The listing builds one solid part. Answer for the finished solid, in the listing's coordinates (mm). A direction names the side the tool comes from. Give positions to 0.01 mm unless a question says otherwise; leave off trailing zeros. Loops run counter-clockwise (first coordinate to the right, second up) from the corner with the lowest first, then second, coordinate; pieces in that order, holes last. Notation, with made-up numbers: M -9.75,84 L 22.25,84 A13 ccw 22.25,94 Z; hole C 43.25,-14 d10. An arc over 180 degrees is marked long. Return JSON: item names as keys, results as strings.
Autodesk Inventor part; units mm, degrees
ref_plane "YZ Plane" through (0, 0, 0) normal (1, 0, 0) x (0, 1, 0)
ref_plane "XZ Plane" through (0, 0, 0) normal (0, 1, 0) x (-1, 0, 0)
ref_plane "XY Plane" through (0, 0, 0) normal (0, 0, 1) x (1, 0, 0)
sketch "Sketch4" plane through (0, 0, 0) normal (0, 1, 0) x (-1, 0, 0)
  line L0 (0, 0) -> (13, 0)
  line L1 (13, 0) -> (13, -13)
  line L2 (13, -13) -> (8.925, -13)
  line L3 (8.925, -13) -> (8.925, -22.5)
  line L4 (8.925, -22.5) -> (1.425, -22.5)
  line L5 (1.425, -22.5) -> (1.425, -13)
  line L6 (1.425, -13) -> (0, -13)
  line L7 (0, -13) -> (0, 0)
  dimension "d17" = 13
  dimension "d18" = 13
  dimension "d19" = 7.5
  dimension "d20" = 1.425
  dimension "d21" = 9.5
extrude "Extrusion2" add sketch "Sketch4" along normal blind 8
sketch "Sketch5" plane through (0, 8, 0) normal (0, 1, 0) x (1, 0, 0)
  line L0 (-8.925, 15) -> (-6.425, 15)
  line L1 (-6.425, 15) -> (-6.425, 20.5)
  line L2 (-6.425, 20.5) -> (-8.925, 20.5)
  line L3 (-8.925, 20.5) -> (-8.925, 15)
  line L4 (-1.425, 22.5) -> (-8.925, 22.5)
  line L5 (-8.925, 22.5) -> (-8.925, 13)
  point P0 (0, 0)
  dimension "d24" = 5.5
  dimension "d25" = 2.5
  dimension "d26" = 2
extrude "Extrusion3" cut sketch "Sketch5" against normal through all
sketch "Sketch6" plane through (0, 8, 0) normal (0, 1, 0) x (1, 0, 0)
  circle A0 centre (-6.5, 6.5) radius 4
  line L0 (-13, 0) -> (0, 0)
  line L1 (0, 0) -> (0, 13)
  dimension "d29" = 8
  dimension "d30" = 6.5
  dimension "d31" = 6.5
extrude "Extrusion4" cut sketch "Sketch6" against normal through all
sketch "Sketch7" plane through (0, 8, 0) normal (0, 1, 0) x (1, 0, 0)
  line L0 (-4.425, 8.5) -> (-3.425, 8.5)
  line L1 (-3.425, 8.5) -> (-3.425, 22.5)
  line L2 (-3.425, 22.5) -> (-4.425, 22.5)
  line L3 (-4.425, 22.5) -> (-4.425, 8.5)
  line L4 (-1.425, 22.5) -> (-8.925, 22.5)
  line L5 (-1.425, 13) -> (-1.425, 22.5)
  point P0 (0, 0)
  dimension "d34" = 1
  dimension "d35" = 14
  dimension "d36" = 2
extrude "Extrusion5" cut sketch "Sketch7" against normal through all
sketch "Sketch8" plane through (-1.425, 0, -13) normal (1, 0, 0) x (0, 0, -1)
  circle A0 centre (4.75, 4) radius 1.65
  line L0 (0, 0) -> (9.5, 0)
  line L1 (9.5, 0) -> (9.5, 8)
  point P0 (-13, 0)
  dimension "d39" = 3.3
  dimension "d40" = 4
  dimension "d41" = 4.75
extrude "Extrusion6" cut sketch "Sketch8" against normal through all
fillet "Fillet1" radius 2 4 edges at (-13, 4, -13) (-13, 4, 0) (0, 4, 0) (0, 4, -13)
properties part number "COLLIER"
(1) Straight lines are drawn through the part: line 1 along Z through (x, y) = (-6.5, 1); line 2 along Y through (x, z) = (-5.1, -17.75); line 3 along X through (y, z) = (3.5, -10.75) (3 decimals). For each, find the intervals that lie inside material, in ascending order.
Values follow:
{"line 1": "-22.5 to -20.5, -15 to -10.5, -2.5 to 0", "line 2": "0 to 2.35, 5.65 to 8", "line 3": "-13 to -4.425, -3.425 to 0"}
(2) A tool of negligible diameter and unlimited length cuts with its end or side. For faces 5 (the flat face through (-8.925, 4, -21)), 6 (the flat face through (-3.425, 4.1, -15.7)), 7 (the flat face through (-1.425, 6, -18)), from which of +Z, -Z, +X, -X, +Y, -Y can it reach the whole face along a straight path? Write none if from no direction.
Values follow:
{"face 5": "-Z, -X, +Y, -Y", "face 6": "-Z, +Y, -Y", "face 7": "-Z, +X, +Y, -Y"}
(3) The part is cut by section A-A (z = -17.75). Determine the outline of the cut face in (x, y) (3 decimals).
Values follow:
{"outline": "M -6.425,0 L -4.425,0 L -4.425,2.35 L -6.425,2.35 Z; M -6.425,5.65 L -4.425,5.65 L -4.425,8 L -6.425,8 Z; M -3.425,0 L -1.425,0 L -1.425,2.35 L -3.425,2.35 Z; M -3.425,5.65 L -1.425,5.65 L -1.425,8 L -3.425,8 Z"}
(4) The part is cut by section C-C (z = -13.25). Determine the outline of the cut face in (x, y) (3 decimals), and give its area (3 significant figures).
Values follow:
{"outline": "M -8.925,0 L -4.425,0 L -4.425,8 L -8.925,8 Z; M -3.425,0 L -1.425,0 L -1.425,8 L -3.425,8 Z", "area": "52.0 mm²"}
(5) Given pin 1 (0.6 mm diameter, centred on y = 5, z = -21.5, fed in from -X) (3 decimals); pin 2 (7 mm diameter, centred on x = -6.5, z = -6.5, fed in from -Y); pin 3 (0.6 mm diameter, centred on x = -9.5, y = 4.5, fed in from -Z); pin 4 (4.5 mm diameter, centred on y = 4, z = -17.75, fed in from -X) (3 decimals), each flat-ended and moving along its own axis, determine where each tip first touches the part or whether it passes through.
Values follow:
{"pin 1": "x = -8.925", "pin 2": "through", "pin 3": "z = -13", "pin 4": "x = -6.425"}
(6) Determine the mould class of faces 1 (the cylindrical face through (-0.406, 3.944, -12.292)), 2 (the flat face through (-8, 4, -20.5)), 3 (the cylindrical face through (-2.411, 4.496, -19.324)), 4 (the flat face through (-8.925, 4, -14)) for opening direction Z: released by +Z, released by -Z, zero draft, split by the parting line, or undercut.
Values follow:
{"face 1": "released by -Z", "face 2": "undercut", "face 3": "undercut", "face 4": "zero draft"}
(7) The part is cut by section B-B (y = 4). Determine the outline of the cut face in (x, z) (3 decimals).
Values follow:
{"outline": "M -13,-11 A2 ccw -11,-13 L -8.925,-13 L -8.925,-15 L -6.425,-15 L -6.425,-16.1 L -4.425,-16.1 L -4.425,-9.92 A4 cw long -3.425,-9.058 L -3.425,-16.1 L -1.425,-16.1 L -1.425,-13 A2 ccw 0,-11.084 L 0,-2 A2 ccw -2,0 L -11,0 A2 ccw -13,-2 Z; M -8.925,-22.5 L -4.425,-22.5 L -4.425,-19.4 L -6.425,-19.4 L -6.425,-20.5 L -8.925,-20.5 Z; M -3.425,-22.5 L -1.425,-22.5 L -1.425,-19.4 L -3.425,-19.4 Z"}
(8) The part is cut by section D-D (x = -9.75). Determine the outline of the cut face in (y, z).
Values follow:
{"outline": "M 0,-13 L 8,-13 L 8,-8.83 L 0,-8.83 Z; M 0,-4.17 L 8,-4.17 L 8,0 L 0,0 Z"}
